For this review, use the dimensioned drawing (mm, ordinates from the lowest corner) and the shaded views. A direction names the side the tool comes from. Give positions to 0.01 mm unless a question says otherwise; leave off trailing zeros. Write each loop counter-clockwise with the first axis right and the second up, starting at its lowest first coordinate (ties: lowest second). Pieces come first, ordered by that corner, then holes. Notation, with made-up numbers: M 60,-26.5 L 85,-26.5 A18 cw 85,4.5 Z; hole C -26.75,-16 d10. An arc over 180 degrees is marked long. Answer in a Markdown table with one row per item.
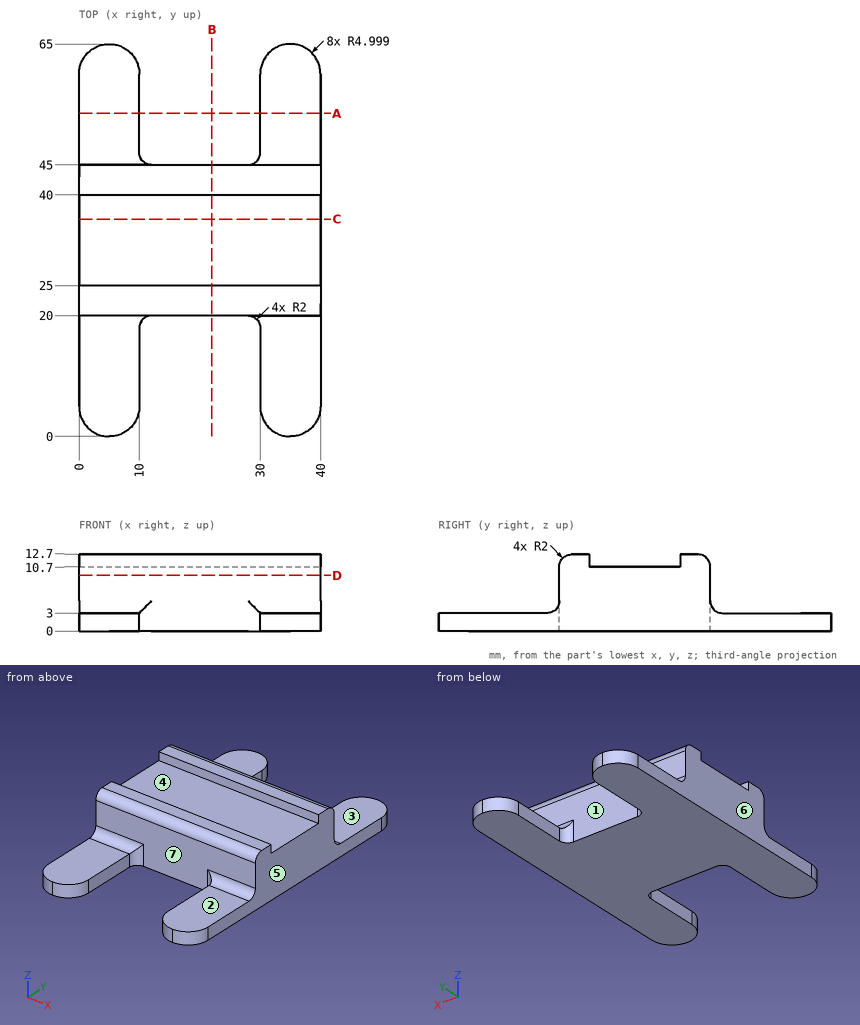
1) Add section B-B (x = 22). Write out the cut boundary in (y, z).
Geometry says:
| item | result |
|---|---|
| outline | M 20,0 L 45,0 L 45,10.7 A2 ccw 43,12.7 L 40,12.7 L 40,10.7 L 25,10.7 L 25,12.7 L 22,12.7 A2 ccw 20,10.7 Z |
2) Add section D-D (z = 9.25). Write out the cut boundary in (x, y).
Geometry says:
| item | result |
|---|---|
| outline | M 0,20 L 40,20 L 40,45 L 0,45 Z |
3) Add section A-A (y = 53.5). Write out the cut boundary in (x, z), and give its area (3 significant figures).
Geometry says:
| item | result |
|---|---|
| outline | M 0,0 L 10,0 L 10,3 L 0,3 Z; M 30,0 L 40,0 L 40,3 L 30,3 Z |
| area | 60.0 mm^2 |
4) For the marked faces 1, 2, 3 and 4, list the 3-axis set-ups (+Z, -Z, +X, -X, +Y, -Y) from which the entire face can be reached by the end or side of a thin tool; tool diameter is ignored.
Geometry says:
| item | result |
|---|---|
| face 1 | +Z, +Y |
| face 2 | +Z, +X, -X, -Y |
| face 3 | +Z, +X, -X, +Y |
| face 4 | +Z, +X, -X |
5) Insertion check: P1, Ø1.5, axis at y = 13, z = 2, coming from the -X side; P2, Ø1, axis at x = 17, y = 37.5, coming from the +Z side; P3, Ø5, axis at x = 35, y = 52.5, coming from the +Z side; P4, Ø6, axis at x = 15.5, z = 10.5, coming from the +Y side. Each pin has a flat end and moves straight along its axis. Give the tip position at first contact, or say it passes through.
Geometry says:
| item | result |
|---|---|
| P1 | x = 0 |
| P2 | z = 10.7 |
| P3 | z = 3 |
| P4 | y = 45 |
6) Add section C-C (y = 36). Write out the cut boundary in (x, z).
Geometry says:
| item | result |
|---|---|
| outline | M 0,0 L 40,0 L 40,10.7 L 0,10.7 Z |
7) The part is to be moulded in two halves that separate along X. For the marked faces 5, 6 and 7, say which applies: released by +X, released by -X, zero draft, split by the parting line, or undercut.
Geometry says:
| item | result |
|---|---|
| face 5 | released by +X |
| face 6 | released by -X |
| face 7 | undercut |
8) To check wall thickness, follow probe 1 along Z at (x, y) = (2, 4.5); probe 2 along X at (y, z) = (60, 2.5); probe 3 along Y at (x, z) = (16.5, 6.5). State the ranges of each line that lie inside material, in increasing order. Write a range as [from, to].
Geometry says:
| item | result |
|---|---|
| probe 1 | [0, 3] |
| probe 2 | [0, 10], [30, 40] |
| probe 3 | [20, 45] |
